Autodesk Inventor part; units mm, degrees
ref_plane "YZ Plane" through (0, 0, 0) normal (1, 0, 0) x (0, 1, 0)
ref_plane "XZ Plane" through (0, 0, 0) normal (0, 1, 0) x (-1, 0, 0)
ref_plane "XY Plane" through (0, 0, 0) normal (0, 0, 1) x (1, 0, 0)
sketch "Sketch1" plane through (0, 0, 0) normal (0, 1, 0) x (-1, 0, 0)
  line L0 (21.65, 21.65) -> (-21.65, 21.65)
  line L1 (-21.65, 21.65) -> (-21.65, -21.65)
  line L2 (-21.65, -21.65) -> (21.65, -21.65)
  line L3 (21.65, -21.65) -> (21.65, 21.65)
  line L4 (21.65, 21.65) -> (-21.65, -21.65) construction
  line L5 (-21.65, 21.65) -> (21.65, -21.65) construction
  line L6 (22.65, 22.65) -> (-22.65, 22.65)
  line L7 (-22.65, 22.65) -> (-22.65, -22.65)
  line L8 (-22.65, -22.65) -> (22.65, -22.65)
  line L9 (22.65, -22.65) -> (22.65, 22.65)
  line L10 (22.65, 22.65) -> (-22.65, -22.65) construction
  line L11 (-22.65, 22.65) -> (22.65, -22.65) construction
  arc A0 (15.65, 18.15) -> (18.15, 15.65) centre (18.15, 18.15) ccw
  circle A1 centre (18.15, 18.15) radius 1.5
  line L12 (25, 0) -> (-31, 0) construction
  line L13 (0, 28) -> (0, -33) construction
  line L14 (15.65, 18.15) -> (15.65, 21.65)
  line L15 (18.15, 15.65) -> (21.65, 15.65)
  arc A2 (18.15, -15.65) -> (15.65, -18.15) centre (18.15, -18.15) ccw
  circle A3 centre (18.15, -18.15) radius 1.5
  line L16 (15.65, -18.15) -> (15.65, -21.65)
  line L17 (18.15, -15.65) -> (21.65, -15.65)
  arc A4 (-18.15, 15.65) -> (-15.65, 18.15) centre (-18.15, 18.15) ccw
  circle A5 centre (-18.15, 18.15) radius 1.5
  line L18 (-15.65, 18.15) -> (-15.65, 21.65)
  line L19 (-18.15, 15.65) -> (-21.65, 15.65)
  circle A6 centre (-18.15, -18.15) radius 1.5
  line L20 (-18.15, -15.65) -> (-21.65, -15.65)
  line L21 (-15.65, -18.15) -> (-15.65, -21.65)
  arc A7 (-15.65, -18.15) -> (-18.15, -15.65) centre (-18.15, -18.15) ccw
  line L22 (28.5, 22.65) -> (-28.5, 22.65)
  line L23 (-28.5, 22.65) -> (-28.5, -22.65)
  line L24 (-28.5, -22.65) -> (28.5, -22.65)
  line L25 (28.5, -22.65) -> (28.5, 22.65)
  line L26 (28.5, 22.65) -> (-28.5, -22.65) construction
  line L27 (-28.5, 22.65) -> (28.5, -22.65) construction
  line L28 (24.65, 18.15) -> (24.65, -18.15) construction
  line L29 (23.05, 18.15) -> (23.05, -18.15)
  line L30 (26.25, -18.15) -> (26.25, 18.15)
  arc A8 (26.25, 18.15) -> (23.05, 18.15) centre (24.65, 18.15) ccw
  arc A9 (23.05, -18.15) -> (26.25, -18.15) centre (24.65, -18.15) ccw
  line L31 (-24.65, 18.15) -> (-24.65, -18.15) construction
  line L32 (-23.05, 18.15) -> (-23.05, -18.15)
  line L33 (-26.25, -18.15) -> (-26.25, 18.15)
  arc A10 (-23.05, 18.15) -> (-26.25, 18.15) centre (-24.65, 18.15) ccw
  arc A11 (-26.25, -18.15) -> (-23.05, -18.15) centre (-24.65, -18.15) ccw
  point P0 (0, 0)
  point P1 (24.65, 0)
  point P2 (-25, 0)
  point P3 (-24.65, 0)
  point P4 (22.65, 22.65)
  point P5 (22.65, -22.65)
  point P6 (-22.65, -22.65)
  dimension "d0" = 43.3
  dimension "d1" = 43.3
  dimension "d2" = 45.3
  dimension "d3" = 45.3
  dimension "d4" = 5
  dimension "d5" = 3.5
  dimension "d6" = 3.5
  dimension "d7" = 3
  dimension "d14" = 3
  dimension "d15" = 57
  dimension "d16" = 3.2
  dimension "d17" = 2
  dimension "d20" = 45.3
extrude "Extrusion1" add sketch "Sketch1" along normal blind 10 contours L9 L8 L7 L6
extrude "Extrusion2" add sketch "Sketch1" along normal blind 2 contours L14 A0 L15 L3 L17 A2 L16 L2 L21 A7 L20 L1 L19 A4 L18 L0
extrude "Extrusion3" add sketch "Sketch1" along normal blind 5 contours L3 L15 A0 L14 L0 | L18 A4 L19 L1 L0 | L3 L2 L16 A2 L17 | L20 A7 L21 L2 L1
extrude "Extrusion4" add sketch "Sketch1" along normal blind 2 contours L22 L25 L24 L9 | L7 L24 L23 L22
sketch "Sketch2" plane through (-21.65, 10, -21.65) normal (0, 0, 1) x (1, 0, 0)
  line L0 (37.3, -8) -> (37.3, -5)
  line L1 (0, 0) -> (43.3, 0)
  line L2 (32.3, -8) -> (11, -8)
  line L3 (6, -3) -> (6, 0)
  line L4 (6, 0) -> (37.3, 0)
  line L5 (37.3, 0) -> (37.3, -3)
  arc A0 (6, -3) -> (11, -8) centre (11, -3) ccw
  arc A1 (32.3, -8) -> (37.3, -3) centre (32.3, -3) ccw
  point P0 (21.65, -10)
  point P1 (6, -8)
  point P2 (37.3, -5)
  dimension "d23" = 5
extrude "Extrusion5" cut sketch "Sketch2" against normal blind 2
sketch "Sketch3" plane through (21.65, 10, -21.65) normal (-1, 0, 0) x (0, 0, 1)
  line L0 (6, -8) -> (37.3, -8)
  line L1 (8, -8) -> (16, -8)
  line L2 (18, -6) -> (18, 0)
  line L3 (18, 0) -> (6, 0)
  line L4 (6, 0) -> (6, -6)
  arc A0 (6, -6) -> (8, -8) centre (8, -6) ccw
  arc A1 (16, -8) -> (18, -6) centre (16, -6) ccw
  point P0 (21.65, -10)
  dimension "d24" = 2
extrude "Extrusion6" cut sketch "Sketch3" against normal blind 2
sketch "Sketch4" plane through (-21.65, 10, 21.65) normal (1, 0, 0) x (0, 0, -1)
  line L0 (37.3, -8) -> (37.3, -5)
  line L1 (44.3, 0) -> (-1, 0)
  line L2 (35.3, -8) -> (27.3, -8)
  line L3 (25.3, -6) -> (25.3, 0)
  line L4 (25.3, 0) -> (37.3, 0)
  line L5 (37.3, 0) -> (37.3, -6)
  arc A0 (25.3, -6) -> (27.3, -8) centre (27.3, -6) ccw
  arc A1 (35.3, -8) -> (37.3, -6) centre (35.3, -6) ccw
  point P0 (21.65, -10)
  dimension "d27" = 12
  dimension "d28" = 2
extrude "Extrusion7" cut sketch "Sketch4" against normal blind 2
properties part number "Mounting L298N_3DPrint"
Read the model definition and answer for the solid it produces. Units are mm, in the model's axes. A direction names the side the tool comes from. Coordinates: 2 decimals unless noted, no trailing zeros. Write each loop counter-clockwise with the first axis right and the second up, starting at its lowest first coordinate (ties: lowest second). Pieces come first, ordered by that corner, then holes. Notation, with made-up numbers: (31, 16.5) -> (84, 16.5) arc R13 cw to (84, 34.5) -> close; hole circle Ø3 at (21.5, -32). An arc over 180 degrees is marked (long way). Return JSON: item names as keys, results as strings.
(1) For a pull along Z with two mould halves and no side action, classify faces 1 (the flat face through (-19.3, 5, 19.4)), 2 (the flat face through (-22, 10, -20)), 3 (the flat face through (0, 5, 22.65)), 4 (the cylindrical face through (24.61, 0.99, -19.75)) as pulls with the +Z half, pulls with the -Z half, needs draft (parallel to the pull), parting line crosses it, or undercut.
Answers below:
{"face 1": "undercut", "face 2": "needs draft", "face 3": "pulls with the +Z half", "face 4": "undercut"}
(2) The part is cut by section A-A on x = 24.65. Give the vertices of the cut face in (y, z), then the cut area to 3 significant figures.
Answers below:
{"outline": "(0, -22.65) -> (2, -22.65) -> (2, -19.75) -> (0, -19.75) -> close; (0, 19.75) -> (2, 19.75) -> (2, 22.65) -> (0, 22.65) -> close", "area": "11.6 mm^2"}
(3) The part is cut by section B-B on y = 1. Give the vertices of the cut face in (x, z), then the cut area to 3 significant figures.
Answers below:
{"outline": "(-28.5, -22.65) -> (28.5, -22.65) -> (28.5, 22.65) -> (-28.5, 22.65) -> close; hole (-26.25, -18.15) arc R1.6 ccw to (-23.05, -18.15) -> (-23.05, 18.15) arc R1.6 ccw to (-26.25, 18.15) -> close; hole circle Ø3 at (-18.15, -18.15); hole circle Ø3 at (-18.15, 18.15); hole circle Ø3 at (18.15, -18.15); hole circle Ø3 at (18.15, 18.15); hole (23.05, -18.15) arc R1.6 ccw to (26.25, -18.15) -> (26.25, 18.15) arc R1.6 ccw to (23.05, 18.15) -> close", "area": "2,310 mm^2"}
(4) Consider line 1 along Z through (x, y) = (-18.15, 3.95); line 2 along Z through (x, y) = (18.15, 1.15). Determine where each line is inside the solid, lowest interval first. Write a range as from..to.
Answers below:
{"line 1": "-22.65..-19.65, -16.65..-15.65, 15.65..16.65, 19.65..22.65", "line 2": "-22.65..-19.65, -16.65..16.65, 19.65..22.65"}
(5) The part is cut by section C-C on z = 3.5. Give the vertices of the cut face in (x, y).
Answers below:
{"outline": "(-28.5, 0) -> (-26.25, 0) -> (-26.25, 2) -> (-28.5, 2) -> close; (-23.05, 0) -> (23.05, 0) -> (23.05, 2) -> (22.65, 2) -> (22.65, 10) -> (21.65, 10) -> (21.65, 2) -> (-21.65, 2) -> (-21.65, 10) -> (-22.65, 10) -> (-22.65, 2) -> (-23.05, 2) -> close; (26.25, 0) -> (28.5, 0) -> (28.5, 2) -> (26.25, 2) -> close"}
(6) Which of the six approach directions +Z, -Z, +X, -X, +Y, -Y give full straight-line access (tool end or side, diameter ignored) to faces 5 (the flat face through (20, 3, 15.65)), 6 (the cylindrical face through (24.69, 0.99, 19.75)), 7 (the cylindrical face through (-22.14, 2.6, -4.22))?
Answers below:
{"face 5": "+Y", "face 6": "+Y, -Y", "face 7": "+X, -X, +Y"}
(7) Each of these flat-tipped pins is pushed along its axis until it touches: P1, Ø1, axis at x = 1.5, z = -18, coming from the +Y side; P2, Ø4, axis at y = 6.5, z = 5.5, coming from the +X side; P3, Ø2.5, axis at y = 5.5, z = 8.5, coming from the -X side. Where does it stop, or does it pass through?
Answers below:
{"P1": "y = 2", "P2": "x = 22.65", "P3": "x = -22.65"}
(8) The part is cut by section D-D on x = -7. Give the vertices of the cut face in (y, z), then the cut area to 3 significant figures.
Answers below:
{"outline": "(0, -22.65) -> (2, -22.65) -> (2, 21.65) -> (10, 21.65) -> (10, 22.65) -> (0, 22.65) -> close", "area": "98.6 mm^2"}
